Autodesk Inventor part; units mm, degrees
ref_plane "YZ Plane" through (0, 0, 0) normal (1, 0, 0) x (0, 1, 0)
ref_plane "XZ Plane" through (0, 0, 0) normal (0, 1, 0) x (-1, 0, 0)
ref_plane "XY Plane" through (0, 0, 0) normal (0, 0, 1) x (1, 0, 0)
sketch "Sketch1" plane through (0, 0, 0) normal (0, 1, 0) x (-1, 0, 0)
  line L0 (9.0067, 0) -> (4.5033, -7.8)
  line L1 (4.5033, -7.8) -> (-4.5033, -7.8)
  line L2 (-4.5033, -7.8) -> (-9.0067, 0)
  line L3 (-9.0067, 0) -> (-4.5033, 7.8)
  line L4 (-4.5033, 7.8) -> (4.5033, 7.8)
  line L5 (4.5033, 7.8) -> (9.0067, 0)
  point P0 (0, 0)
  point P1 (0, 0)
  dimension "d0" = 15.6
extrude "Extrusion1" add sketch "Sketch1" along normal blind 4
sketch "Sketch2" plane through (0, 4, 0) normal (0, 1, 0) x (1, 0, 0)
  line L0 (-4.5033, -7.8) -> (4.5033, -7.8)
  line L1 (4.5033, -7.8) -> (9.0067, 0)
  line L2 (9.0067, 0) -> (4.5033, 7.8)
  line L3 (4.5033, 7.8) -> (-4.5033, 7.8)
  line L4 (-4.5033, 7.8) -> (-9.0067, 0)
  line L5 (-9.0067, 0) -> (-4.5033, -7.8)
  circle A0 centre (0, 0) radius 9.0067
extrude "Extrusion2" add sketch "Sketch2" along normal blind 1.2
sketch "Sketch3" plane through (0, 0, 0) normal (1, 0, 0) x (0, 1, 0)
  line L0 (-4, 0.0705) -> (1.2, 9.0772)
  line L1 (-4, 0.0705) -> (6.4, 0.0705) construction
  line L2 (1.2, 9.0772) -> (-4, 9.0772)
  line L3 (-4, 9.0772) -> (-4, 0.0705)
  line L4 (0, 13.9781) -> (0, -14.7276)
  line L5 (13.4115, 0) -> (-11.0286, 0)
  point P0 (0, 0)
  dimension "d5" = 60
  dimension "d6" = 5.2
  dimension "d7" = 4
revolve "Revolution1" cut sketch "Sketch3" angle 360 about axis through (0, 13.4115, 0) along (0, -1, 0)
sketch "Sketch4" plane through (0, 5.2, 0) normal (0, 1, 0) x (1, 0, 0)
  point P0 (0, 0)
  point P1 (0, 0)
hole "Hole1" at (0, 5.2, 0) direction (0, -1, 0) diameter 10.106 end through all
properties part number "Cable Gland Lock Nut RS 822-9791"
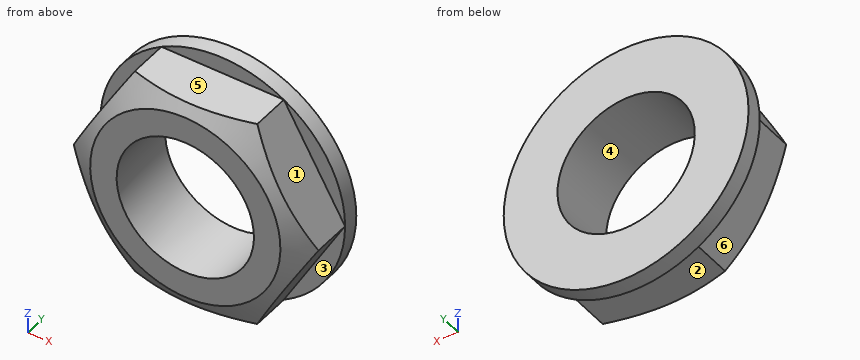
The model under review builds one solid part; all positions refer to its coordinate system, in mm. Face numbers are marked on the shaded views. A direction names the side the tool comes from. Round coordinates to 2 decimals unless told otherwise and drop trailing zeros. Write each loop counter-clockwise with the first axis right and the second up, starting at its lowest first coordinate (ties: lowest second). Pieces come first, ordered by that corner, then holes. Notation, with made-up numbers: (-28, 85.5) - (11, 85.5) arc R14 ccw to (11, 96.5) - close; hole circle Ø3 at (-9.5, -1.75). An arc over 180 degrees is marked (long way). Answer as CSV lines item,"result". Start each with the question number.
(1) To check wall thickness, follow line 1 (Z direction, x = 0, y = 1.85); line 2 (Z direction, x = 0, y = 4.15); line 3 (X direction, y = 3.6, z = 4.5). State the ranges of each line that lie inside material, in increasing order.
(2) For pin 1 Ø1.1 at (x, y) = (1.5, 2.5) entering from -Z; pin 2 Ø1.4 at (x, z) = (7, -5.5) entering from -Y; pin 3 Ø1.5 at (x, y) = (-6, 4.5) entering from +Z, all flat-tipped, find the tip position at first contact; note any pin that passes through.
(3) For the marked faces 1, 2 and 3, list the 3-axis set-ups (+Z, -Z, +X, -X, +Y, -Y) from which the entire face can be reached by the end or side of a thin tool; tool diameter is ignored.
(4) We need section A-A on x = 0. State the section outline as (y, z) points.
(5) Draft analysis for pull direction Z (two halves, no side actions). For the marked faces 4, 5 and 6, state which applies: pulls with the +Z half, pulls with the -Z half, needs draft (parallel to the pull), parting line crosses it, or undercut.
(6) We need section B-B on y = 2.6. State the section outline as (x, z) points.
Worked answers:
1,line 1,"-7.8 to -5.05, 5.05 to 7.8"
1,line 2,"-9.01 to -5.05, 5.05 to 9.01"
1,line 3,"-6.41 to -2.3, 2.3 to 6.41"
2,pin 1,"z = -7.8"
2,pin 2,"y = 4"
2,pin 3,"z = 7.32"
3,face 1,"+Z, +X, -Y"
3,face 2,"-Z, +X, -X, -Y"
3,face 3,"-Z, +X, -Y"
4,outline,"(0, -7) - (0.46, -7.8) - (4, -7.8) - (4, -9.01) - (5.2, -9.01) - (5.2, -5.05) - (0, -5.05) - close; (0, 5.05) - (5.2, 5.05) - (5.2, 9.01) - (4, 9.01) - (4, 7.8) - (0.46, 7.8) - (0, 7) - close"
5,face 4,"undercut"
5,face 5,"pulls with the +Z half"
5,face 6,"pulls with the -Z half"
6,outline,"(-9.01, 0) - (-4.5, -7.8) - (4.5, -7.8) - (9.01, 0) - (4.5, 7.8) - (-4.5, 7.8) - close; hole circle Ø10.11 at (0, 0)"
